```python
from build123d import *

# Parameters (mm, degrees)
SKETCH1_W            = 56
SKETCH1_H            = 53
BOSS_EXTRUDE1_DEPTH  = 2
BOSS_EXTRUDE2_DEPTH  = 4
SKETCH3_W            = 56
SKETCH3_H            = 2
BOSS_EXTRUDE3_DEPTH  = 6
SKETCH4_W            = 2.5
SKETCH4_H            = 6
BOSS_EXTRUDE4_DEPTH  = 4
SKETCH5_W            = 2.5
SKETCH5_H            = 6
BOSS_EXTRUDE5_DEPTH  = 4
SKETCH6_W            = 6
SKETCH6_H            = 6
BOSS_EXTRUDE6_DEPTH  = 1.5
SKETCH7_W            = 6
SKETCH7_H            = 6
BOSS_EXTRUDE7_DEPTH  = 1.5
SKETCH8_W            = 2
SKETCH8_H            = 4
BOSS_EXTRUDE8_DEPTH  = 2.5
SKETCH9_W            = 2
SKETCH9_H            = 4
BOSS_EXTRUDE9_DEPTH  = 2.5
SKETCH10_W           = 52
SKETCH10_H           = 1
BOSS_EXTRUDE10_DEPTH = 5.5
CUT_EXTRUDE1_DEPTH   = 5.5
SKETCH12_R           = 1.25
CUT_EXTRUDE2_DEPTH   = 15.5
SKETCH13_R           = 1.25
CUT_EXTRUDE3_DEPTH   = 15.5
SKETCH14_W           = 8.5
SKETCH14_H           = 4
BOSS_EXTRUDE11_DEPTH = 2.5
SKETCH15_W           = 8.5
SKETCH15_H           = 4
BOSS_EXTRUDE12_DEPTH = 2.5
SKETCH16_W           = 10.5
SKETCH16_H           = 6
BOSS_EXTRUDE13_DEPTH = 1.5
SKETCH17_W           = 10.5
SKETCH17_H           = 6
BOSS_EXTRUDE14_DEPTH = 1.5
SKETCH18_R           = 1.25
CUT_EXTRUDE4_DEPTH   = 10
SKETCH19_R           = 1.25
CUT_EXTRUDE5_DEPTH   = 10
CHAMFER4_SIZE        = 1


with BuildPart() as part:
    # Sketch1 → Boss-Extrude1 (new body)
    with BuildSketch(Plane(origin=(0, 0, 0), x_dir=(1, 0, 0), z_dir=(0, 1, 0))):
        Rectangle(SKETCH1_W, SKETCH1_H)
    extrude(amount=BOSS_EXTRUDE1_DEPTH)

    # Sketch2 → Boss-Extrude2 (add)
    with BuildSketch(Plane(origin=(0, 2, 0), x_dir=(1, 0, 0), z_dir=(0, 1, 0))):
        Polygon((-26, 26.5), (-28, 26.5), (-28, -23), (-28, -26.5), (-26, -26.5), (26, -26.5), (28, -26.5), (28, -23), (28, 26.5), (26, 26.5), (26, -24.5), (-26, -24.5), align=None)
    extrude(amount=BOSS_EXTRUDE2_DEPTH)

    # Sketch3 → Boss-Extrude3 (add)
    with BuildSketch(Plane(origin=(0, 6, 0), x_dir=(1, 0, 0), z_dir=(0, 1, 0))):
        with Locations((0, -25.5)):
            Rectangle(SKETCH3_W, SKETCH3_H)
    extrude(amount=BOSS_EXTRUDE3_DEPTH)

    # Sketch4 → Boss-Extrude4 (add)
    with BuildSketch(Plane(origin=(0, 2, 0), x_dir=(1, 0, 0), z_dir=(0, 1, 0))):
        with Locations((-24.75, 23.5)):
            Rectangle(SKETCH4_W, SKETCH4_H)
    extrude(amount=BOSS_EXTRUDE4_DEPTH)

    # Sketch5 → Boss-Extrude5 (add)
    with BuildSketch(Plane(origin=(0, 2, 0), x_dir=(1, 0, 0), z_dir=(0, 1, 0))):
        with Locations((24.75, 23.5)):
            Rectangle(SKETCH5_W, SKETCH5_H)
    extrude(amount=BOSS_EXTRUDE5_DEPTH)

    # Sketch6 → Boss-Extrude6 (add)
    with BuildSketch(Plane.ZY.offset(28)):
        with Locations((-23.5, 3)):
            Rectangle(SKETCH6_W, SKETCH6_H)
    extrude(amount=BOSS_EXTRUDE6_DEPTH)

    # Sketch7 → Boss-Extrude7 (add)
    with BuildSketch(Plane(origin=(28, 0, 0), x_dir=(0, 0, -1), z_dir=(1, 0, 0))):
        with Locations((23.5, 3)):
            Rectangle(SKETCH7_W, SKETCH7_H)
    extrude(amount=BOSS_EXTRUDE7_DEPTH)

    # Sketch8 → Boss-Extrude8 (add)
    with BuildSketch(Plane.ZY.offset(-26)):
        with Locations((-0.5, 4)):
            Rectangle(SKETCH8_W, SKETCH8_H)
    extrude(amount=BOSS_EXTRUDE8_DEPTH)

    # Sketch9 → Boss-Extrude9 (add)
    with BuildSketch(Plane(origin=(-26, 0, 0), x_dir=(0, 0, -1), z_dir=(1, 0, 0))):
        with Locations((0.5, 4)):
            Rectangle(SKETCH9_W, SKETCH9_H)
    extrude(amount=BOSS_EXTRUDE9_DEPTH)

    # Sketch10 → Boss-Extrude10 (add)
    with BuildSketch(Plane(origin=(0, 2, 0), x_dir=(1, 0, 0), z_dir=(0, 1, 0))):
        with Locations((0, -8.5)):
            Rectangle(SKETCH10_W, SKETCH10_H)
    extrude(amount=BOSS_EXTRUDE10_DEPTH)

    # Sketch11 → Cut-Extrude1 (cut)
    with BuildSketch(Plane.XY.offset(26.5)):
        with BuildLine():
            Line((-24.75, 9.5), (-24.75, 12))
            Line((-24.75, 12), (24.75, 13))
            ThreePointArc((24.75, 13), (23.799038106, 11.162882693), (21.75, 10.878679656))
            Line((21.75, 10.878679656), (21.75, 9.5))
            ThreePointArc((21.75, 9.5), (19.5, 7.25), (17.25, 9.5))
            Line((17.25, 9.5), (17.25, 10.878679656))
            ThreePointArc((17.25, 10.878679656), (16.5, 10.75), (15.75, 10.878679656))
            Line((15.75, 10.878679656), (15.75, 9.5))
            ThreePointArc((15.75, 9.5), (13.5, 7.25), (11.25, 9.5))
            Line((11.25, 9.5), (11.25, 10.878679656))
            ThreePointArc((11.25, 10.878679656), (10.5, 10.75), (9.75, 10.878679656))
            Line((9.75, 10.878679656), (9.75, 9.5))
            ThreePointArc((9.75, 9.5), (7.5, 7.25), (5.25, 9.5))
            Line((5.25, 9.5), (5.25, 10.878679656))
            ThreePointArc((5.25, 10.878679656), (4.5, 10.75), (3.75, 10.878679656))
            Line((3.75, 10.878679656), (3.75, 9.5))
            ThreePointArc((3.75, 9.5), (1.5, 7.25), (-0.75, 9.5))
            Line((-0.75, 9.5), (-0.75, 10.878679656))
            ThreePointArc((-0.75, 10.878679656), (-1.5, 10.75), (-2.25, 10.878679656))
            Line((-2.25, 10.878679656), (-2.25, 9.5))
            ThreePointArc((-2.25, 9.5), (-4.5, 7.25), (-6.75, 9.5))
            Line((-6.75, 9.5), (-6.75, 10.878679656))
            ThreePointArc((-6.75, 10.878679656), (-7.5, 10.75), (-8.25, 10.878679656))
            Line((-8.25, 10.878679656), (-8.25, 9.5))
            ThreePointArc((-8.25, 9.5), (-10.5, 7.25), (-12.75, 9.5))
            Line((-12.75, 9.5), (-12.75, 10.878679656))
            ThreePointArc((-12.75, 10.878679656), (-13.5, 10.75), (-14.25, 10.878679656))
            Line((-14.25, 10.878679656), (-14.25, 9.5))
            ThreePointArc((-14.25, 9.5), (-16.5, 7.25), (-18.75, 9.5))
            Line((-18.75, 9.5), (-18.75, 10.878679656))
            ThreePointArc((-18.75, 10.878679656), (-19.5, 10.75), (-20.25, 10.878679656))
            Line((-20.25, 10.878679656), (-20.25, 9.5))
            ThreePointArc((-20.25, 9.5), (-22.5, 7.25), (-24.75, 9.5))
        make_face()
    extrude(amount=-CUT_EXTRUDE1_DEPTH, mode=Mode.SUBTRACT)

    # Sketch12 → Cut-Extrude2 (cut)
    with BuildSketch(Plane(origin=(0, 6, 0), x_dir=(1, 0, 0), z_dir=(0, 1, 0))):
        with Locations(Location((26.5, 23.5, 0), (0, 0, 270))):
            Circle(SKETCH12_R)
    extrude(amount=-CUT_EXTRUDE2_DEPTH, mode=Mode.SUBTRACT)

    # Sketch13 → Cut-Extrude3 (cut)
    with BuildSketch(Plane(origin=(0, 6, 0), x_dir=(1, 0, 0), z_dir=(0, 1, 0))):
        with Locations(Location((-26.5, 23.5, 0), (0, 0, 270))):
            Circle(SKETCH13_R)
    extrude(amount=-CUT_EXTRUDE3_DEPTH, mode=Mode.SUBTRACT)

    # Sketch14 → Boss-Extrude11 (add)
    with BuildSketch(Plane(origin=(-26, 0, 0), x_dir=(0, 0, -1), z_dir=(1, 0, 0))):
        with Locations((-4.75, 4)):
            Rectangle(SKETCH14_W, SKETCH14_H)
    extrude(amount=BOSS_EXTRUDE11_DEPTH)

    # Sketch15 → Boss-Extrude12 (add)
    with BuildSketch(Plane.ZY.offset(-26)):
        with Locations((4.75, 4)):
            Rectangle(SKETCH15_W, SKETCH15_H)
    extrude(amount=BOSS_EXTRUDE12_DEPTH)

    # Sketch16 → Boss-Extrude13 (add)
    with BuildSketch(Plane.ZY.offset(28)):
        with Locations((3.75, 3)):
            Rectangle(SKETCH16_W, SKETCH16_H)
    extrude(amount=BOSS_EXTRUDE13_DEPTH)

    # Sketch17 → Boss-Extrude14 (add)
    with BuildSketch(Plane(origin=(28, 0, 0), x_dir=(0, 0, -1), z_dir=(1, 0, 0))):
        with Locations((-3.75, 3)):
            Rectangle(SKETCH17_W, SKETCH17_H)
    extrude(amount=BOSS_EXTRUDE14_DEPTH)

    # Sketch18 → Cut-Extrude4 (cut)
    with BuildSketch(Plane(origin=(0, 6, 0), x_dir=(1, 0, 0), z_dir=(0, 1, 0))):
        with Locations(Location((26.5, -3.5, 0), (0, 0, 270))):
            Circle(SKETCH18_R)
    extrude(amount=-CUT_EXTRUDE4_DEPTH, mode=Mode.SUBTRACT)

    # Sketch19 → Cut-Extrude5 (cut)
    with BuildSketch(Plane(origin=(0, 6, 0), x_dir=(1, 0, 0), z_dir=(0, 1, 0))):
        with Locations(Location((-26.5, -3.5, 0), (0, 0, 270))):
            Circle(SKETCH19_R)
    extrude(amount=-CUT_EXTRUDE5_DEPTH, mode=Mode.SUBTRACT)

    # Chamfer4
    chamfer4_edges = [part.edges().sort_by_distance(p)[0] for p in [
        (-28, 0, 17.75),
        (28, 0, -11),
        (0, 0, 26.5),
        (28, 0, 17.75),
        (-28, 0, -11),
    ]]
    chamfer(chamfer4_edges, length=CHAMFER4_SIZE)


solid = part.part
```
The model under review builds one solid part; all positions refer to its coordinate system, in mm. A direction names the side the tool comes from. Give positions to 0.01 mm unless a question says otherwise; leave off trailing zeros. Loops run counter-clockwise (first coordinate to the right, second up) from the corner with the lowest first, then second, coordinate; pieces in that order, holes last. Notation, with made-up numbers: (59, 88) -> (88, 88) arc R16 cw to (88, 102) -> close; hole circle Ø1 at (-15, 7). An arc over 180 degrees is marked (long way). Use CSV: the item, a comma, the result in double quotes.
1. Consider section B-B, the plane x = 1.5. Write out the cut boundary in (y, z).
Result:
outline,"(0, -26.5) -> (2, -26.5) -> (2, 8) -> (7.5, 8) -> (7.5, 9) -> (2, 9) -> (2, 24.5) -> (7.25, 24.5) -> (7.25, 26.5) -> (1, 26.5) -> (0, 25.5) -> close"
2. Consider section D-D, the plane z = -13. Write out the cut boundary in (x, y), then the cut area to 3 significant figures.
Result:
outline,"(-28, 1) -> (-27, 0) -> (27, 0) -> (28, 1) -> (28, 6) -> (26, 6) -> (26, 2) -> (-26, 2) -> (-26, 6) -> (-28, 6) -> close"
area,"127 mm²"
3. For P1, Ø0.7, axis at y = 10, z = 26, coming from the -X side; P2, Ø2, axis at y = 3, z = 16, coming from the +X side; P3, Ø6.5, axis at x = 26.5, z = -6, coming from the +Y side, all flat-tipped, find the tip position at first contact; note any pin that passes through.
Result:
P1,"stops at x = -28"
P2,"stops at x = 28"
P3,"stops at y = 6"
4. To check wall thickness, follow probe 1 along Z at (x, y) = (-24.5, 5.5); probe 2 along X at (y, z) = (3.75, 3.5); probe 3 along X at (y, z) = (1.85, -23.5). State the ranges of each line that lie inside material, in increasing order. Write a range as from..to.
Result:
probe 1,"z = -26.5..-20.5, -1.5..9, 24.5..26.5"
probe 2,"x = -29.5..-27.75, -25.25..-23.5, 23.5..25.25, 27.75..29.5"
probe 3,"x = -29.5..-27.75, -25.25..25.25, 27.75..29.5"
5. The part is to be moulded in two halves that separate along Z. For faces 1 (the face through (-26.12, 3.04, 4.69)), 2 (the face through (23.5, 4, 3)), 3 (the face through (-0.4, 1.6, -26.5)), say which applies: +Z half, -Z half, draft (parallel to the pull), parting line (faces both ways), or undercut.
Result:
face 1,"undercut"
face 2,"draft"
face 3,"-Z half"
6. Consider section C-C, the plane y = 2.75. Count the separate pieces of the cut face and the enclosed holes in it, then the cut area to 3 significant figures.
Result:
separate pieces,"1"
enclosed holes,"5"
area,"475 mm²"
7. Consider section A-A, the plane z = 3.5. Write out the cut boundary in (x, y), then the cut area to 3 significant figures.
Result:
outline,"(-29.5, 0) -> (-27.75, 0) -> (-27.75, 6) -> (-29.5, 6) -> close; (-25.25, 0) -> (25.25, 0) -> (25.25, 6) -> (23.5, 6) -> (23.5, 2) -> (-23.5, 2) -> (-23.5, 6) -> (-25.25, 6) -> close; (27.75, 0) -> (29.5, 0) -> (29.5, 6) -> (27.75, 6) -> close"
area,"136 mm²"
8. Machinability: for faces 4 (the face through (11.25, 10, 26)), 5 (the face through (29.5, 3, 4)), 6 (the face through (0, 2, 17)), 7 (the face through (23.5, 4, -23)), 8 (the face through (-4.45, 7.25, 25.51)), which of the approach directions +Z, -Z, +X, -X, +Y, -Y give a long, thin tool a straight path to every point of the face, cutting with its end or side? Answer none if there is none.
Result:
face 4,"+Z, -Z, +Y"
face 5,"+Z, -Z, +X, +Y, -Y"
face 6,"+Y"
face 7,"-Z, +Y"
face 8,"+Z, +Y"
